```python
from build123d import *

# Parameters (mm, degrees)
CROQUIS1_W                       = 394
CROQUIS1_H                       = 127
CROQUIS1_R                       = 15
SALIENTE_EXTRUIR1_DEPTH          = 4.7625
CROQUIS2_R                       = 3
CORTAR_EXTRUIR1_DEPTH            = 365.565057851
CROQUIS3_R                       = 3
CORTAR_EXTRUIR2_DEPTH            = 365.565057851
MATRIZC1_COUNT                   = 4
BRIDA_DE_ARISTA1_STRIP_W         = 39.05
BRIDA_DE_ARISTA1_STRIP_H         = 4.7625
BRIDA_DE_ARISTA1_STRIP_CUT_DEPTH = 394
BRIDA_DE_ARISTA1_DEPTH           = 394
CORTAR_EXTRUIR3_DEPTH            = 369.084229491
CROQUIS15_R                      = 7.5
CORTAR_EXTRUIR4_DEPTH            = 369.084229491
CROQUIS16_R                      = 8
CORTAR_EXTRUIR5_DEPTH            = 369.084229491


# Sheet-metal steps are written as plain solids
with BuildPart() as part:
    # Croquis1 → Saliente-Extruir1 (new body)
    with BuildSketch(Plane.XY):
        with Locations((157, 23.5)):
            Rectangle(CROQUIS1_W, CROQUIS1_H)
        with Locations(Location((0, 0, 0), (0, 0, 180))):
            Circle(CROQUIS1_R, mode=Mode.SUBTRACT)
        with Locations(Location((314, 30, 0), (0, 0, 180))):
            Circle(CROQUIS1_R, mode=Mode.SUBTRACT)
    extrude(amount=SALIENTE_EXTRUIR1_DEPTH)

    # Croquis2 → Cortar-Extruir1 (cut, through all)
    with BuildSketch(Plane.XY.offset(4.7625)):
        with Locations((0, 27.597586589)):
            Circle(CROQUIS2_R)
        with Locations((27.597586589, 0)):
            Circle(CROQUIS2_R)
        with Locations((0, -27.597586589)):
            Circle(CROQUIS2_R)
        with Locations((-27.597586589, 0)):
            Circle(CROQUIS2_R)
    extrude(amount=-CORTAR_EXTRUIR1_DEPTH, mode=Mode.SUBTRACT)

    # Croquis3 → Cortar-Extruir2 (cut, through all)
    with BuildSketch(Plane.XY.offset(4.7625)):
        with Locations((314, 57.6)):
            Circle(CROQUIS3_R)
    cortar_extruir2 = extrude(amount=-CORTAR_EXTRUIR2_DEPTH, mode=Mode.SUBTRACT)

    # MatrizC1: Cortar-Extruir2 ×4 about axis
    matrizc1_axis = Axis((314, 30, 0), (0, 0, 1))
    for i in range(1, MATRIZC1_COUNT):
        add(cortar_extruir2.rotate(matrizc1_axis, i * 360 / MATRIZC1_COUNT), mode=Mode.SUBTRACT)

    # Brida de arista1 strip (across the edge) → Brida de arista1 strip cut (cut)
    with BuildSketch(Plane(origin=(354, 87, 4.7625), x_dir=(0, -1, 0), z_dir=(-1, 0, 0))):
        with Locations((-4.7625, -2.38125)):
            Rectangle(BRIDA_DE_ARISTA1_STRIP_W, BRIDA_DE_ARISTA1_STRIP_H)
    extrude(amount=BRIDA_DE_ARISTA1_STRIP_CUT_DEPTH, mode=Mode.SUBTRACT)

    # Brida de arista1 section (across the edge) → Brida de arista1 (add)
    with BuildSketch(Plane(origin=(354, 87, 4.7625), x_dir=(0, -1, 0), z_dir=(-1, 0, 0))):
        with BuildLine():
            Line((0, 10), (0, 46.2375))
            Line((0, 46.2375), (4.7625, 46.2375))
            Line((4.7625, 46.2375), (4.7625, 10))
            ThreePointArc((4.7625, 10), (7.691432188, 2.928932188), (14.7625, 0))
            Line((14.7625, 0), (14.7625, -4.7625))
            ThreePointArc((14.7625, -4.7625), (4.323836143, -0.438663857), (0, 10))
        make_face()
    extrude(amount=BRIDA_DE_ARISTA1_DEPTH)

    # Croquis14 → Cortar-Extruir3 (cut, through all)
    with BuildSketch(Plane(origin=(0, 0, 0), x_dir=(-1, 0, 0), z_dir=(0, 0, -1))):
        with BuildLine():
            Line((-7, 59), (-161, 59))
            ThreePointArc((-161, 59), (-166, 64), (-161, 69))
            Line((-161, 69), (-7, 69))
            ThreePointArc((-7, 69), (-2, 64), (-7, 59))
        make_face()
    extrude(amount=-CORTAR_EXTRUIR3_DEPTH, mode=Mode.SUBTRACT)

    # Croquis15 → Cortar-Extruir4 (cut, through all)
    with BuildSketch(Plane(origin=(0, 0, 0), x_dir=(-1, 0, 0), z_dir=(0, 0, -1))):
        with Locations((-44, 32)):
            Circle(CROQUIS15_R)
    extrude(amount=-CORTAR_EXTRUIR4_DEPTH, mode=Mode.SUBTRACT)

    # Croquis16 → Cortar-Extruir5 (cut, through all)
    with BuildSketch(Plane(origin=(0, 0, 0), x_dir=(-1, 0, 0), z_dir=(0, 0, -1))):
        with Locations((-276, 64)):
            Circle(CROQUIS16_R)
    extrude(amount=-CORTAR_EXTRUIR5_DEPTH, mode=Mode.SUBTRACT)


solid = part.part
```
CAD build for the part. Positions are in the model's coordinates, mm. A direction names the side the tool comes from. Round coordinates to 2 decimals unless told otherwise and drop trailing zeros. Loops run counter-clockwise (first coordinate to the right, second up) from the corner with the lowest first, then second, coordinate; pieces in that order, holes last. Notation, with made-up numbers: M -2.5,33 L 41.5,33 A24 ccw 41.5,51 Z; hole C 10.25,-24.75 d6. An arc over 180 degrees is marked long. Use a Markdown table: item, result. Add a question column.
(1) Pull direction X, two halves, no side cores. Call faces 3 (the face through (40.539, 25.346, 2.348)), 4 (the face through (159.76, 82.56, 4.21)), 5 (the face through (-40, 42, 3)): +X half, -X half, draft (parallel to the pull), parting line (faces both ways), or undercut.
(2) Flat gauge pins, fed straight in: pin 1 (5 mm diameter, centred on x = 0, y = -27.6, fed in from -Z); pin 2 (18 mm diameter, centred on x = 105.5, z = 31, fed in from -Y); pin 3 (5 mm diameter, centred on x = 88, z = 2.5, fed in from +Y); pin 4 (21 mm diameter, centred on x = 276, y = 64, fed in from +Z). Where does each tip first touch, or does it go through?
(3) Cut at D-D (x = 195.5). Give the cut face in (y, z) (1 decimal).
(4) Drill centre lines: line 1 (X direction, y = 57, z = 1); line 2 (Y direction, x = 0, z = 2.8); line 3 (Y direction, x = 0, z = 3.6). Where is each one in solid material? Low to high.
(5) Which spindle directions (+Z, -Z, +X, -X, +Y, -Y) get a long thin tool onto all of the face, cutting with end or side? Do faces 1 (the face through (154, 17, 4.762)), 2 (the face through (271.699, 70.746, 2.348)). Say none if no direction does.
(6) Cut at B-B (x = 141.5). Give the cut face in (y, z) (1 decimal), and give its area (3 significant figures).
(7) Cut at A-A (y = 21). Give the cut face in (x, z).
(8) Cut at C-C (y = 64). Give the cut face in (x, z).
Geometry says:
| question | item | result |
|---|---|---|
| 1 | face 3 | undercut |
| 1 | face 4 | draft |
| 1 | face 5 | -X half |
| 2 | pin 1 | passes through |
| 2 | pin 2 | stops at y = 82.24 |
| 2 | pin 3 | stops at y = 83.31 |
| 2 | pin 4 | stops at z = 5.02 |
| 3 | outline | M -40,0 L 72.2,0 A14.8 ccw 87,14.8 L 87,51 L 82.2,51 L 82.2,14.8 A10 cw 72.2,4.8 L -40,4.8 Z |
| 4 | line 1 | x = -40 to 272.13, 279.87 to 311.06, 316.94 to 354 |
| 4 | line 2 | y = -40 to -30.6, -24.6 to -15, 15 to 24.6, 30.6 to 80.89 |
| 4 | line 3 | y = -40 to -30.6, -24.6 to -15, 15 to 24.6, 30.6 to 81.9 |
| 5 | face 1 | +Z, +X, -X, -Y |
| 5 | face 2 | +Z, -Z |
| 6 | outline | M -40,0 L 59,0 L 59,4.8 L -40,4.8 Z; M 69,0 L 72.2,0 A14.8 ccw 87,14.8 L 87,51 L 82.2,51 L 82.2,14.8 A10 cw 72.2,4.8 L 69,4.8 Z |
| 6 | area | 752 mm² |
| 7 | outline | M -40,0 L 302,0 L 302,4.76 L -40,4.76 Z; M 326,0 L 354,0 L 354,4.76 L 326,4.76 Z |
| 8 | outline | M -40,0 L 2,0 L 2,4.76 L -40,4.76 Z; M 166,0 L 268,0 L 268,4.76 L 166,4.76 Z; M 284,0 L 354,0 L 354,4.76 L 284,4.76 Z |
